Geometry: final body of the model. Coordinates: model frame, mm. A direction names the side the tool comes from. Round coordinates to 2 decimals unless told otherwise and drop trailing zeros. Loops run counter-clockwise (first coordinate to the right, second up) from the corner with the lowest first, then second, coordinate; pieces in that order, holes last. Notation, with made-up numbers: (-18.5, 59) - (32.5, 59) arc R19 cw to (32.5, 70) - close; hole circle Ø3 at (56.5, -19.75). An arc over 180 degrees is marked (long way). Write item = value, one per line. Start each with the question number.
Item 1: Section A-A (x = 0). Return loops of the section in (y, z).
Item 2: Section B-B (z = 10). Return loops of the section in (x, y).
Item 3: Section D-D (y = 2.35). Count the separate pieces of the cut face and the enclosed holes in it, plus the area to 3 significant figures.
Item 4: Access query for faces 1 (the cylindrical face through (-119.26, 2.54, 0.37)), 2 (the cylindrical face through (94.218, 2.535, 10.62)). Directions: +Z, -Z, +X, -X, +Y, -Y. A direction counts if a zero-diameter tool reaches every point of the face in a straight line with its end or side. Return the directions, or none.
Item 5: Line query: line 1 (Z direction, x = -55.5, y = 2.35); line 2 (X direction, y = 1.8, z = 29.5); line 3 (X direction, y = 4.05, z = -16). Output: solid intervals per line, ascending. Write a range as from..to.
Item 6: First-contact query: pin 1 (2.5 mm diameter, centred on x = 72, y = 2, fed in from -Z). Flat tip, straight axial feed; report the tip coordinate or a pass-through.
Item 7: Draft query along Z for faces 3 (the flat face through (2, 2, 50)), 4 (the cylindrical face through (56.582, 2.465, -37.937)), 5 (the flat face through (-120, 2, 22)). Return one class per face: pulls with the +Z half, pulls with the -Z half, needs draft (parallel to the pull), parting line crosses it, or undercut.
Item 8: Section C-C (x = 76.5). Return loops of the section in (y, z).
from build123d import *

# Parameters (mm, degrees)
SKETCH_1_R          = 20
SKETCH_1_R_2        = 2.6
EXTRUDE_1_DEPTH     = 5
CUT_EXTRUDE_2_DEPTH = 5
FILLET_1_R          = 10
SKETCH_3_R          = 1.6
CUT_EXTRUDE_3_DEPTH = 131.096118313
SKETCH_4_R          = 1.6
CUT_EXTRUDE_4_DEPTH = 131.096118313


with BuildPart() as part:
    # ｽｹｯﾁ1 → ﾎﾞｽ - 押し出し1 (new body)
    with BuildSketch(Plane(origin=(0, 0, 0), x_dir=(1, 0, 0), z_dir=(0, 1, 0))):
        Polygon((-120, -50), (-120, 0), (-70, 50), (70, 50), (120, 0), (120, -50), align=None)
        with Locations(Location((0, 0, 0), (0, 0, 270))):
            Circle(SKETCH_1_R, mode=Mode.SUBTRACT)
        with Locations(Location((-110, -35, 0), (0, 0, 270))):
            Circle(SKETCH_1_R_2, mode=Mode.SUBTRACT)
        with Locations(Location((-110, -5, 0), (0, 0, 270))):
            Circle(SKETCH_1_R_2, mode=Mode.SUBTRACT)
        with Locations(Location((-55, 40, 0), (0, 0, 270))):
            Circle(SKETCH_1_R_2, mode=Mode.SUBTRACT)
        with Locations(Location((0, 40, 0), (0, 0, 270))):
            Circle(SKETCH_1_R_2, mode=Mode.SUBTRACT)
        with Locations(Location((110, -35, 0), (0, 0, 90))):
            Circle(SKETCH_1_R_2, mode=Mode.SUBTRACT)
        with Locations(Location((110, -5, 0), (0, 0, 90))):
            Circle(SKETCH_1_R_2, mode=Mode.SUBTRACT)
        with Locations(Location((55, 40, 0), (0, 0, 90))):
            Circle(SKETCH_1_R_2, mode=Mode.SUBTRACT)
    extrude(amount=EXTRUDE_1_DEPTH)

    # ｽｹｯﾁ2 → ｶｯﾄ - 押し出し2 (cut)
    with BuildSketch(Plane(origin=(0, 5, 0), x_dir=(1, 0, 0), z_dir=(0, 1, 0))):
        with BuildLine():
            Line((-62.573593129, 22.071067812), (-92.071067812, -7.426406871))
            ThreePointArc((-92.071067812, -7.426406871), (-94.238795325, -10.670640359), (-95, -14.497474683))
            Line((-95, -14.497474683), (-95, -25))
            ThreePointArc((-95, -25), (-92.071067812, -32.071067812), (-85, -35))
            Line((-85, -35), (-45, -35))
            ThreePointArc((-45, -35), (-37.928932188, -32.071067812), (-35, -25))
            Line((-35, -25), (-35, 15))
            ThreePointArc((-35, 15), (-37.928932188, 22.071067812), (-45, 25))
            Line((-45, 25), (-55.502525317, 25))
            ThreePointArc((-55.502525317, 25), (-59.329359641, 24.238795325), (-62.573593129, 22.071067812))
        make_face()
        with BuildLine():
            Line((35, -25), (35, 15))
            ThreePointArc((35, 15), (37.928932188, 22.071067812), (45, 25))
            Line((45, 25), (55.502525317, 25))
            ThreePointArc((55.502525317, 25), (59.329359641, 24.238795325), (62.573593129, 22.071067812))
            Line((62.573593129, 22.071067812), (92.071067812, -7.426406871))
            ThreePointArc((92.071067812, -7.426406871), (94.238795325, -10.670640359), (95, -14.497474683))
            Line((95, -14.497474683), (95, -25))
            ThreePointArc((95, -25), (92.071067812, -32.071067812), (85, -35))
            Line((85, -35), (45, -35))
            ThreePointArc((45, -35), (37.928932188, -32.071067812), (35, -25))
        make_face()
    extrude(amount=-CUT_EXTRUDE_2_DEPTH, mode=Mode.SUBTRACT)

    # ﾌｨﾚｯﾄ1
    fillet_1_edges = [part.edges().sort_by_distance(p)[0] for p in [
        (-120, 2.5, 50),
        (-120, 2.5, 0),
        (-70, 2.5, -50),
        (70, 2.5, -50),
        (120, 2.5, 0),
        (120, 2.5, 50),
    ]]
    fillet(fillet_1_edges, radius=FILLET_1_R)

    # ｽｹｯﾁ3 → ｶｯﾄ - 押し出し3 (cut, through all)
    with BuildSketch(Plane(origin=(0, 5, 0), x_dir=(1, 0, 0), z_dir=(0, 1, 0))):
        with Locations(Location((-20, 20, 0), (0, 0, 270))):
            Circle(SKETCH_3_R)
        with Locations(Location((20, 20, 0), (0, 0, 270))):
            Circle(SKETCH_3_R)
        with Locations(Location((20, -20, 0), (0, 0, 270))):
            Circle(SKETCH_3_R)
        with Locations(Location((-20, -20, 0), (0, 0, 270))):
            Circle(SKETCH_3_R)
    extrude(amount=-CUT_EXTRUDE_3_DEPTH, mode=Mode.SUBTRACT)

    # ｽｹｯﾁ4 → ｶｯﾄ - 押し出し4 (cut, through all)
    with BuildSketch(Plane(origin=(0, 5, 0), x_dir=(1, 0, 0), z_dir=(0, 1, 0))):
        with Locations(Location((-35, 40, 0), (0, 0, 270))):
            Circle(SKETCH_4_R)
        with Locations(Location((35, 40, 0), (0, 0, 90))):
            Circle(SKETCH_4_R)
    extrude(amount=-CUT_EXTRUDE_4_DEPTH, mode=Mode.SUBTRACT)


solid = part.part
Taken from the geometry:
q1.outline = (0, -50) - (5, -50) - (5, -42.6) - (0, -42.6) - close; (0, -37.4) - (5, -37.4) - (5, -20) - (0, -20) - close; (0, 20) - (5, 20) - (5, 50) - (0, 50) - close
q2.outline = (-120, 0) - (-93.93, 0) - (-93.93, 5) - (-120, 5) - close; (-35, 0) - (-17.32, 0) - (-17.32, 5) - (-35, 5) - close; (17.32, 0) - (35, 0) - (35, 5) - (17.32, 5) - close; (93.93, 0) - (120, 0) - (120, 5) - (93.93, 5) - close
q3.separate_pieces = 1
q3.enclosed_holes = 16
q3.area = 14,200 mm^2
q4.face_1 = -Z, -X, +Y, -Y
q4.face_2 = +Y, -Y
q5.line_1 = -50..-42.55, -37.45..-25, 35..50
q5.line_2 = -120..-93.93, -36.07..36.07, 93.93..120
q5.line_3 = -104..-68.64, -35.05..-12, 12..35.05, 68.64..104
q6.pin_1 = -48.72
q7.face_3 = pulls with the +Z half
q7.face_4 = undercut
q7.face_5 = needs draft
q8.outline = (0, -43.5) - (5, -43.5) - (5, -8.14) - (0, -8.14) - close; (0, 35) - (5, 35) - (5, 50) - (0, 50) - close
